Source: CAD feature listing. Evaluate the final solid. Frame: model axes, mm. Face numbers are marked on the shaded views. A direction names the side the tool comes from. Round coordinates to 2 decimals unless told otherwise and drop trailing zeros. Write each loop counter-clockwise with the first axis right and the second up, starting at its lowest first coordinate (ties: lowest second). Pieces come first, ordered by that corner, then holes. Notation, with made-up numbers: (5, 72) - (48, 72) arc R28 cw to (48, 110) - close; hole circle Ø7 at (22, 17.5). An arc over 180 degrees is marked (long way). Write item = value, one per line. Start each with the question number.
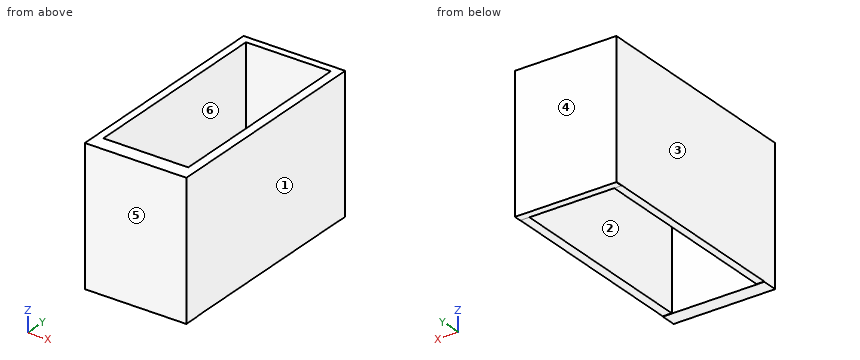
```python
from build123d import *

# Parameters (mm, degrees)
F0_W     = 169.4771945477
F0_H     = 226.4695465565
F1_DEPTH = 25.4
F3_W     = 345.577955246
F3_H     = 225.8900702
F4_DEPTH = 12.8757357597
F2_W     = 345.919251442
F2_H     = 225.8651852608
F5_DEPTH = 15.0449182838
F7_DEPTH = 12.402491644


with BuildPart() as f1:
    # F0 (on Front) → F1 (new body)
    with BuildSketch(Plane.XZ):
        Rectangle(F0_W, F0_H)
    extrude(amount=F1_DEPTH)

    # F3 (on face) → F4 (join)
    with BuildSketch(Plane(origin=(-84.7385972738, 0, 0), x_dir=(0, -1, 0), z_dir=(-1, 0, 0))):
        with Locations((-172.788977623, 0.2897381783)):
            Rectangle(F3_W, F3_H)
    extrude(amount=-F4_DEPTH)

    # F2 (on face) → F5 (join)
    with BuildSketch(Plane.YZ.offset(84.7385972738)):
        with Locations((172.959625721, 0.3021806479)):
            Rectangle(F2_W, F2_H)
    extrude(amount=-F5_DEPTH)

    # F6 (on face) → F7 (join)
    with BuildSketch(Plane(origin=(0, 345.919251442, 0), x_dir=(-1, 0, 0), z_dir=(0, 1, 0))):
        Polygon((84.5447480679, 113.2347732782), (-69.69367899, 113.2347732782), (-69.69367899, -112.6304119825), (-84.7385972738, -112.6304119825), (-84.7385972738, -113.1013929844), (84.5447480679, -113.1013929844), align=None)
    extrude(amount=-F7_DEPTH)


solid = f1.part
```
(1) Pull-direction query (Y, two-part tool) for the marked faces 3, 4, 5 and 6; classes: +Y half, -Y half, draft (parallel to the pull), parting line (faces both ways), or undercut.
(2) Reachability of the marked faces 1 and 2 from +Z, -Z, +X, -X, +Y, -Y: full face, straight path, thin tool, end or side. Return the list, or none.
(3) Ray query, L1, parallel to X at y = 150, z = -75; L2, parallel to Y at x = 5.5, z = 8; L3, parallel to Z at x = 71, y = 313.5. Return the intervals inside material, ascending. Write a range as from..to.
(4) Contact query for flat-ended pins moving along their axis: P1, Ø6.5, axis at x = -81.5, y = 106, coming from the -Z side; P2, Ø16.5, axis at x = 75, y = 158.5, coming from the -Z side; P3, Ø6, axis at x = 29, y = 338.5, coming from the -Z side. Output: stop coordinate, or through.
(5) Section B-B (x = 14). Return the cut outline in (y, z).
(6) Section A-A (y = 74). Return the cut outline in (x, z).
(7) Section C-C (z = -91). Return the cut outline in (x, y), plus the area to 3 significant figures.
Solution:
q1.face_3 = draft
q1.face_4 = +Y half
q1.face_5 = -Y half
q1.face_6 = undercut
q2.face_1 = +Z, -Z, +X, +Y, -Y
q2.face_2 = +Z, -Z
q3.L1 = -84.74..-71.86, 69.69..84.74
q3.L2 = -25.4..0, 333.52..345.92
q3.L3 = -112.63..113.23
q4.P1 = -112.66
q4.P2 = -112.63
q4.P3 = -113.1
q5.outline = (-25.4, -113.23) - (0, -113.23) - (0, 113.23) - (-25.4, 113.23) - close; (333.52, -113.1) - (345.92, -113.1) - (345.92, 113.23) - (333.52, 113.23) - close
q6.outline = (-84.74, -112.66) - (-71.86, -112.66) - (-71.86, 113.23) - (-84.74, 113.23) - close; (69.69, -112.63) - (84.74, -112.63) - (84.74, 113.23) - (69.69, 113.23) - close
q7.outline = (-84.74, -25.4) - (84.74, -25.4) - (84.74, 345.92) - (-84.54, 345.92) - (-84.54, 345.58) - (-84.74, 345.58) - close; hole (-71.86, 0) - (69.69, 0) - (69.69, 333.52) - (-71.86, 333.52) - close
q7.area = 15,700 mm^2
